from build123d import *

# Parameters (mm, degrees)
SKETCH1_W           = 14
SKETCH1_H           = 14
SKETCH1_W_2         = 13.96
SKETCH1_H_2         = 13.96
SKETCH1_W_3         = 17.83
SKETCH1_H_3         = 34.365
SKETCH1_W_4         = 16.8
SKETCH1_H_4         = 14.955
BOSS_EXTRUDE2_DEPTH = 4
SKETCH3_W           = 14
SKETCH3_H           = 16
CUT_EXTRUDE1_DEPTH  = 2.5
SKETCH6_W           = 145
SKETCH6_H           = 81.124541
BOSS_EXTRUDE3_DEPTH = 7
SKETCH12_R          = 0.8
CUT_EXTRUDE5_DEPTH  = 6
SKETCH13_W          = 17.97
SKETCH13_H          = 46.826347
CUT_EXTRUDE6_DEPTH  = 6
SKETCH14_W          = 16.8
SKETCH14_H          = 14.955
CUT_EXTRUDE8_DEPTH  = 4.6
SKETCH15_R          = 4
CUT_EXTRUDE9_DEPTH  = 10
SKETCH16_R          = 12
CUT_EXTRUDE10_DEPTH = 1
SKETCH20_W          = 145
SKETCH20_H          = 81.124541
SKETCH20_W_2        = 130
SKETCH20_H_2        = 66.1
BOSS_EXTRUDE5_DEPTH = 1
SKETCH21_W          = 145
SKETCH21_H          = 34.866824831
CUT_EXTRUDE11_DEPTH = 18
FILLET1_R           = 3
SKETCH27_W          = 17.97
SKETCH27_H          = 5.776347
CUT_EXTRUDE13_DEPTH = 2
CUT_EXTRUDE14_START = -2
CUT_EXTRUDE14_DEPTH = 2
SKETCH28_W          = 17.854591413
SKETCH28_H          = 5
CUT_EXTRUDE15_DEPTH = 2


# Read off the part's stored shape, not the designer's step: Cut-Extrude14
with BuildPart() as part:
    # Sketch1 → Boss-Extrude2 (new body)
    with BuildSketch(Plane(origin=(0, 0, 0), x_dir=(1, 0, 0), z_dir=(0, 1, 0))):
        Polygon((0, 0), (109.34, 0), (130, 0), (130, 66.1), (0, 66.1), align=None)
        with Locations((51.87, 10.55)):
            Rectangle(SKETCH1_W, SKETCH1_H, mode=Mode.SUBTRACT)
        with Locations((32.81, 10.55)):
            Rectangle(SKETCH1_W, SKETCH1_H, mode=Mode.SUBTRACT)
        with Locations((32.81, 29.6)):
            Rectangle(SKETCH1_W, SKETCH1_H, mode=Mode.SUBTRACT)
        with Locations((32.79, 48.63)):
            Rectangle(SKETCH1_W_2, SKETCH1_H_2, mode=Mode.SUBTRACT)
        with Locations((13.145, 42.2325)):
            Rectangle(SKETCH1_W_3, SKETCH1_H_3, mode=Mode.SUBTRACT)
        with Locations((13.75, 10.55)):
            Rectangle(SKETCH1_W, SKETCH1_H, mode=Mode.SUBTRACT)
        with Locations((51.87, 29.6)):
            Rectangle(SKETCH1_W, SKETCH1_H, mode=Mode.SUBTRACT)
        with Locations((70.93, 10.55)):
            Rectangle(SKETCH1_W, SKETCH1_H, mode=Mode.SUBTRACT)
        with Locations((89.99, 10.55)):
            Rectangle(SKETCH1_W, SKETCH1_H, mode=Mode.SUBTRACT)
        with Locations((117.74, 14.4625)):
            Rectangle(SKETCH1_W_4, SKETCH1_H_4, mode=Mode.SUBTRACT)
        with Locations((70.93, 29.6)):
            Rectangle(SKETCH1_W, SKETCH1_H, mode=Mode.SUBTRACT)
        with Locations((89.99, 29.6)):
            Rectangle(SKETCH1_W, SKETCH1_H, mode=Mode.SUBTRACT)
        with Locations((51.87, 48.65)):
            Rectangle(SKETCH1_W, SKETCH1_H, mode=Mode.SUBTRACT)
        with Locations((70.93, 48.65)):
            Rectangle(SKETCH1_W, SKETCH1_H, mode=Mode.SUBTRACT)
        with Locations((89.99, 48.65)):
            Rectangle(SKETCH1_W, SKETCH1_H, mode=Mode.SUBTRACT)
        with Locations((117.74, 44.7175)):
            Rectangle(SKETCH1_W_4, SKETCH1_H_4, mode=Mode.SUBTRACT)
    extrude(amount=BOSS_EXTRUDE2_DEPTH)

    # Sketch3 → Cut-Extrude1 (cut)
    with BuildSketch(Plane(origin=(0, 0, 0), x_dir=(1, 0, 0), z_dir=(0, 1, 0))):
        with Locations((89.99, 29.6)):
            Rectangle(SKETCH3_W, SKETCH3_H)
        with Locations((70.93, 29.6)):
            Rectangle(SKETCH3_W, SKETCH3_H)
        with Locations((89.99, 48.65)):
            Rectangle(SKETCH3_W, SKETCH3_H)
        with Locations((70.93, 48.65)):
            Rectangle(SKETCH3_W, SKETCH3_H)
        with Locations((51.87, 48.65)):
            Rectangle(SKETCH3_W, SKETCH3_H)
        with Locations((32.81, 48.65)):
            Rectangle(SKETCH3_W, SKETCH3_H)
        with Locations((32.81, 29.650197757)):
            Rectangle(SKETCH3_W, SKETCH3_H)
        with Locations((51.87, 29.6)):
            Rectangle(SKETCH3_W, SKETCH3_H)
        with Locations((13.75, 10.55)):
            Rectangle(SKETCH3_W, SKETCH3_H)
        with Locations((32.81, 10.55)):
            Rectangle(SKETCH3_W, SKETCH3_H)
        with Locations((51.87, 10.55)):
            Rectangle(SKETCH3_W, SKETCH3_H)
        with Locations((70.93, 10.55)):
            Rectangle(SKETCH3_W, SKETCH3_H)
        with Locations((89.99, 10.55)):
            Rectangle(SKETCH3_W, SKETCH3_H)
    extrude(amount=CUT_EXTRUDE1_DEPTH, mode=Mode.SUBTRACT)

    # Sketch6 → Boss-Extrude3 (add)
    with BuildSketch(Plane(origin=(0, 0, 0), x_dir=(-1, 0, 0), z_dir=(0, -1, 0))):
        with Locations((-65, 33.3140765)):
            Rectangle(SKETCH6_W, SKETCH6_H)
        Polygon((-99.99, 58.61), (-39.77, 58.61), (-22.81, 58.61), (-22.81, 53.222321133), (-22.81, 20.55), (-3.75, 20.55), (-3.75, 12.496372948), (-3.75, 0.461789698), (-20.75, 0.461789698), (-99.99, 0.461789698), align=None, mode=Mode.SUBTRACT)
    extrude(amount=-BOSS_EXTRUDE3_DEPTH)

    # Sketch12 → Cut-Extrude5 (cut)
    with BuildSketch(Plane(origin=(0, 0, 0), x_dir=(-1, 0, 0), z_dir=(0, -1, 0))):
        with BuildLine():
            ThreePointArc((-1.45, 63.85), (-1.684314575, 64.415685425), (-2.25, 64.65))
            Line((-2.25, 64.65), (-2.25, 63.85))
            Line((-2.25, 63.85), (-1.45, 63.85))
        make_face()
        with BuildLine():
            Line((-2.25, 63.85), (-2.25, 64.65))
            ThreePointArc((-2.25, 64.65), (-2.815685425, 63.284314575), (-1.45, 63.85))
            Line((-1.45, 63.85), (-2.25, 63.85))
        make_face()
        with BuildLine():
            ThreePointArc((-1.45, 2.25), (-2.815685425, 2.815685425), (-2.25, 1.45))
            Line((-2.25, 1.45), (-2.25, 2.25))
            Line((-2.25, 2.25), (-1.45, 2.25))
        make_face()
        with BuildLine():
            Line((-2.25, 2.25), (-2.25, 1.45))
            ThreePointArc((-2.25, 1.45), (-1.684314575, 1.684314575), (-1.45, 2.25))
            Line((-1.45, 2.25), (-2.25, 2.25))
        make_face()
        with BuildLine():
            ThreePointArc((-128.55, 2.25), (-128.315685425, 1.684314575), (-127.75, 1.45))
            Line((-127.75, 1.45), (-127.75, 2.25))
            Line((-127.75, 2.25), (-128.55, 2.25))
        make_face()
        with BuildLine():
            Line((-127.75, 2.25), (-127.75, 1.45))
            ThreePointArc((-127.75, 1.45), (-127.184314575, 1.684314575), (-126.95, 2.25))
            ThreePointArc((-126.95, 2.25), (-127.75, 3.05), (-128.55, 2.25))
            Line((-128.55, 2.25), (-127.75, 2.25))
        make_face()
        with Locations(Location((-127.75, 63.85, 0), (0, 0, 90))):
            Circle(SKETCH12_R)
    extrude(amount=-CUT_EXTRUDE5_DEPTH, mode=Mode.SUBTRACT)

    # Sketch13 → Cut-Extrude6 (cut)
    with BuildSketch(Plane.XZ):
        with Locations((13.215, -48.4631735)):
            Rectangle(SKETCH13_W, SKETCH13_H)
    extrude(amount=-CUT_EXTRUDE6_DEPTH, mode=Mode.SUBTRACT)

    # Sketch14 → Cut-Extrude8 (cut)
    with BuildSketch(Plane.XZ):
        with Locations((117.74, -14.4625)):
            Rectangle(SKETCH14_W, SKETCH14_H)
        with Locations((117.74, -44.7175)):
            Rectangle(SKETCH14_W, SKETCH14_H)
    extrude(amount=-CUT_EXTRUDE8_DEPTH, mode=Mode.SUBTRACT)

    # Sketch15 → Cut-Extrude9 (cut)
    with BuildSketch(Plane.XZ):
        with Locations(Location((117.74, -44.7175, 0), (0, 0, 270))):
            Circle(SKETCH15_R)
        with Locations(Location((117.74, -14.4625, 0), (0, 0, 270))):
            Circle(SKETCH15_R)
    extrude(amount=-CUT_EXTRUDE9_DEPTH, mode=Mode.SUBTRACT)

    # Sketch16 → Cut-Extrude10 (cut)
    with BuildSketch(Plane(origin=(0, 7, 0), x_dir=(1, 0, 0), z_dir=(0, 1, 0))):
        with Locations(Location((117.74, 44.7175, 0), (0, 0, 270))):
            Circle(SKETCH16_R)
        with Locations(Location((117.74, 14.4625, 0), (0, 0, 270))):
            Circle(SKETCH16_R)
    extrude(amount=-CUT_EXTRUDE10_DEPTH, mode=Mode.SUBTRACT)

    # Sketch20 → Boss-Extrude5 (add)
    with BuildSketch(Plane.XZ):
        with Locations((65, -33.3140765)):
            Rectangle(SKETCH20_W, SKETCH20_H)
        with Locations((65, -33.05)):
            Rectangle(SKETCH20_W_2, SKETCH20_H_2, mode=Mode.SUBTRACT)
    extrude(amount=BOSS_EXTRUDE5_DEPTH)

    # Sketch21 → Cut-Extrude11 (cut)
    with BuildSketch(Plane(origin=(0, -1.861896279, 0.228612117), x_dir=(-1, 0, 0), z_dir=(0, 0.9925461516413211, -0.1218693434051548))):
        with Locations((-65, 24.505710134)):
            Rectangle(SKETCH21_W, SKETCH21_H)
    extrude(amount=CUT_EXTRUDE11_DEPTH, mode=Mode.SUBTRACT)

    # Fillet1
    fillet1_edges = [part.edges().sort_by_distance(p)[0] for p in [
        (-7.5, 3, 6.757055756),
        (137.5, 3, 6.757055756),
    ]]
    fillet(fillet1_edges, radius=FILLET1_R)

    # Sketch27 → Cut-Extrude13 (cut)
    with BuildSketch(Plane.XZ):
        with Locations((13.215, -68.9881735)):
            Rectangle(SKETCH27_W, SKETCH27_H)
    extrude(amount=CUT_EXTRUDE13_DEPTH, mode=Mode.SUBTRACT)

    # Cut-Extrude14 outline → Cut-Extrude14 (cut)
    with BuildSketch(Plane(origin=(0, 7, 0), x_dir=(1, 0, 0), z_dir=(0, 1, 0)).offset(CUT_EXTRUDE14_START)):
        Polygon((4.351462148, 71.876347), (9.23, 71.876347), (9.23, 62.876347), (17.321462297, 62.876347), (17.321462297, 71.876347), (22.2, 71.876347), (22.2, 73.876347), (4.351462148, 73.876347), align=None)
    extrude(amount=CUT_EXTRUDE14_DEPTH, mode=Mode.SUBTRACT)

    # Sketch28 → Cut-Extrude15 (cut)
    with BuildSketch(Plane(origin=(0, 0, -73.876347), x_dir=(-1, 0, 0), z_dir=(0, 0, -1))):
        with Locations((-13.272704442, 2.5)):
            Rectangle(SKETCH28_W, SKETCH28_H)
    extrude(amount=-CUT_EXTRUDE15_DEPTH, mode=Mode.SUBTRACT)


solid = part.part
Design review of the part built by this model. Coordinates are the model's own, in mm. A direction names the side the tool comes from. Coordinates: 2 decimals unless noted, no trailing zeros. Use one line per item in the form item = value. Start each with the question number.
(1) Add section A-A on x = 72.5. Give the number of separate pieces and of enclosed holes in the cut face, plus the area to 3 significant figures.
(2) For faces 1 (the flat face through (13, 5, -20.55)), 2 (the flat face through (52, 1, -37.6)), list the 3-axis set-ups (+Z, -Z, +X, -X, +Y, -Y) from which the entire face can be reached by the end or side of a thin tool; tool diameter is ignored.
(3) For probe 1 along Z at (x, y) = (30.5, 1); probe 2 along X at (y, z) = (1, -35.5); probe 3 along Z at (x, y) = (2.25, 2.85), list the stretches that pass through material, from the lowest coordinate up.
(4) Insertion check: pin 1 (6 mm diameter, centred on x = 9.5, z = -51.5, fed in from -Y); pin 2 (0.8 mm diameter, centred on x = 87.5, y = 3, fed in from +Z); pin 3 (1 mm diameter, centred on x = 52, z = -37.5, fed in from +Y). Each pin has a flat end and moves straight along its axis. Give the tip position at first contact, or say it passes through.
Answer block:
q1.separate_pieces = 4
q1.enclosed_holes = 0
q1.area = 222 mm²
q2.face_1 = +Y
q2.face_2 = -Y
q3.probe_1 = -73.88 to -56.65, -40.65 to -37.65, -21.65 to -18.55, -2.55 to 7
q3.probe_2 = -7.5 to 4.23, 22.2 to 25.81, 39.81 to 44.87, 58.87 to 63.93, 77.93 to 82.99, 96.99 to 137.5
q3.probe_3 = -73.88 to -64.65, -63.05 to -3.05, -1.45 to 6.78
q4.pin_1 = 6
q4.pin_2 = 6.81
q4.pin_3 = 4
